Source: CAD feature listing. Evaluate the final solid. Frame: model axes, mm. A direction names the side the tool comes from. Round coordinates to 2 decimals unless told otherwise and drop trailing zeros. Order: outer loops, then holes, each group sorted by start corner. A loop starts at its lowest first (then second) coordinate and runs counter-clockwise, first axis right, second up. Notation, with made-up numbers: M 60.5,57 L 94.5,57 A14 ccw 94.5,79 Z; hole C -36,-16.75 d7. An arc over 180 degrees is marked long. Use CSV: the item, a comma, the result in double quotes. Start each with the question number.
```python
from build123d import *

# Parameters (mm, degrees)
SKETCH1_W           = 24
SKETCH1_H           = 90
BOSS_EXTRUDE1_DEPTH = 20
CUT_EXTRUDE1_DEPTH  = 16
CUT_EXTRUDE8_DEPTH  = 10
FILLET1_R           = 20
SKETCH12_R          = 2.5
CUT_EXTRUDE9_DEPTH  = 18.5
SKETCH13_R          = 4.5
CUT_EXTRUDE10_DEPTH = 16.5
FILLET2_R           = 3
CHAMFER1_SIZE       = 3


with BuildPart() as part:
    # Sketch1 → Boss-Extrude1 (new body)
    with BuildSketch(Plane.XY):
        with Locations((12, 45)):
            Rectangle(SKETCH1_W, SKETCH1_H)
    extrude(amount=-BOSS_EXTRUDE1_DEPTH)

    # Sketch4 → Cut-Extrude1 (cut)
    with BuildSketch(Plane.XY):
        Polygon((20.5, 83), (18.5, 83), (18.5, 61), (19.5, 61), (8, 15), (8, 0), (24, 0), (24, 90), (20.5, 90), align=None)
    extrude(amount=-CUT_EXTRUDE1_DEPTH, mode=Mode.SUBTRACT)

    # Sketch9 → Cut-Extrude8 (cut)
    with BuildSketch(Plane(origin=(0, 0, -20), x_dir=(-1, 0, 0), z_dir=(0, 0, -1))):
        Polygon((-24, 0), (-24, 45), (-8, 15), (-8, 0), align=None)
    extrude(amount=-CUT_EXTRUDE8_DEPTH, mode=Mode.SUBTRACT)

    # Fillet1
    fillet1_edges = [part.edges().sort_by_distance(p)[0] for p in [
        (24, 45, -18),
    ]]
    fillet(fillet1_edges, radius=FILLET1_R)

    # Sketch12 → Cut-Extrude9 (cut)
    with BuildSketch(Plane(origin=(18.5, 0, 0), x_dir=(0, 0, -1), z_dir=(1, 0, 0))):
        with Locations(Location((10, 72, 0), (0, 0, 90))):
            Circle(SKETCH12_R)
        with Locations(Location((10, 7.5, 0), (0, 0, 90))):
            Circle(SKETCH12_R)
    extrude(amount=-CUT_EXTRUDE9_DEPTH, mode=Mode.SUBTRACT)

    # Sketch13 → Cut-Extrude10 (cut)
    with BuildSketch(Plane(origin=(18.5, 0, 0), x_dir=(0, 0, -1), z_dir=(1, 0, 0))):
        with Locations(Location((10, 72, 0), (0, 0, 90))):
            Circle(SKETCH13_R)
        with Locations(Location((10, 7.5, 0), (0, 0, 90))):
            Circle(SKETCH13_R)
    extrude(amount=-CUT_EXTRUDE10_DEPTH, mode=Mode.SUBTRACT)

    # Fillet2
    # the kernel refuses this fillet: 3 mm, written as the material it takes off along each edge
    with BuildSketch(Plane(origin=(0, 90, 7.5), x_dir=(1, 0, 0), z_dir=(0, 0, -1)), Plane(origin=(8, 0, -27.5), x_dir=(0, 1, 0), z_dir=(0, 0, 1)), Plane(origin=(0, 0, 7.5), x_dir=(0, 1, 0), z_dir=(0, 0, -1))) as fillet2_piece_1:
        with BuildLine():
            CenterArc((FILLET2_R, FILLET2_R), FILLET2_R, 180, 90)
            Line((0, FILLET2_R), (-FILLET2_R * 0.02, FILLET2_R))
            Line((-FILLET2_R * 0.02, FILLET2_R), (-FILLET2_R * 0.02, -FILLET2_R * 0.02))
            Line((-FILLET2_R * 0.02, -FILLET2_R * 0.02), (FILLET2_R, -FILLET2_R * 0.02))
            Line((FILLET2_R, -FILLET2_R * 0.02), (FILLET2_R, 0))
        make_face()
    extrude(amount=35, mode=Mode.SUBTRACT)
    with BuildSketch(Plane(origin=(24, 90, -8.5), x_dir=(0, -1, 0), z_dir=(0, 0, -1))) as fillet2_piece_2:
        with BuildLine():
            CenterArc((FILLET2_R, FILLET2_R), FILLET2_R, 180, 90)
            Line((0, FILLET2_R), (-FILLET2_R * 0.02, FILLET2_R))
            Line((-FILLET2_R * 0.02, FILLET2_R), (-FILLET2_R * 0.02, -FILLET2_R * 0.02))
            Line((-FILLET2_R * 0.02, -FILLET2_R * 0.02), (FILLET2_R, -FILLET2_R * 0.02))
            Line((FILLET2_R, -FILLET2_R * 0.02), (FILLET2_R, 0))
        make_face()
    extrude(amount=19, mode=Mode.SUBTRACT)
    with BuildSketch(Plane(origin=(19.5, 61, 6.128837665), x_dir=(-0.24253562503633366, -0.9701425001453317, 0), z_dir=(0, 0, -1))) as fillet2_piece_3:
        with BuildLine():
            CenterArc((2.451535066, 3), FILLET2_R, 222.580014358, 47.419985642)
            Line((0.242535625, 0.9701425), (0.198355636, 0.92954535))
            ThreePointArc((0.198355636, 0.92954535), (0.063059263, 0.499623388), (-0.05820855, 0.014552138))
            Line((-0.05820855, 0.014552138), (0, -0.06))
            Line((0, -0.06), (2.451535066, -0.06))
            Line((2.451535066, -0.06), (2.451535066, 0))
        make_face()
    extrude(amount=22.128837665, mode=Mode.SUBTRACT)

    # Chamfer1
    # the kernel refuses this chamfer: 3 mm, written as the material it takes off along each edge
    with BuildSketch(Plane(origin=(21, 87, -16), x_dir=(1, 0, 0), z_dir=(0, -1, 0))) as chamfer1_piece_1:
        Polygon((3 - CHAMFER1_SIZE, 0), (3, -CHAMFER1_SIZE), (3, 0), align=None)
    revolve(axis=Axis((21, 87, -16), (0, 0, 1)), revolution_arc=90, mode=Mode.SUBTRACT)
    with BuildSketch(Plane(origin=(24, 50, -16), x_dir=(-1, 0, 0), z_dir=(0, 1, 0))) as chamfer1_piece_2:
        Polygon((CHAMFER1_SIZE, 0), (0, -CHAMFER1_SIZE), (0, 0), align=None)
    extrude(amount=37, mode=Mode.SUBTRACT)
    with BuildSketch(Plane(origin=(4.369388723, 8.192603855, -16), x_dir=(0, 0, -1), z_dir=(0.47058823529411764, 0.8823529411764706, 0))) as chamfer1_piece_3_section:
        Polygon((CHAMFER1_SIZE, 0), (0, CHAMFER1_SIZE), (0, 0), align=None)
    chamfer1_piece_3 = extrude(amount=36.715048964, mode=Mode.PRIVATE)
    chamfer1_piece_3 = split(chamfer1_piece_3, bisect_by=Plane(origin=(8, 8.192603855, -16), z_dir=(1, 0, 0)), keep=Keep.TOP, mode=Mode.PRIVATE)
    chamfer1_piece_3 = split(chamfer1_piece_3, bisect_by=Plane(origin=(6.184694361, 7.738777446, -16), z_dir=(0.9701425001453319, -0.24253562503633322, 0)), keep=Keep.TOP, mode=Mode.PRIVATE)
    add(chamfer1_piece_3, mode=Mode.SUBTRACT)
    with BuildSketch(Plane(origin=(4, 50, -16), x_dir=(0.8823529411764705, -0.47058823529411764, 0), z_dir=(-0.47058823529411764, -0.8823529411764705, 0))) as chamfer1_piece_4:
        Polygon((20, -CHAMFER1_SIZE), (20 - CHAMFER1_SIZE, 0), (20, 0), align=None)
    revolve(axis=Axis((4, 50, -16), (0, 0, 1)), revolution_arc=28.072486936, mode=Mode.SUBTRACT)
    with BuildSketch(Plane(origin=(21, 90, -16), x_dir=(0, -1, 0), z_dir=(-1, 0, 0))) as chamfer1_piece_5:
        Polygon((CHAMFER1_SIZE, 0), (0, -CHAMFER1_SIZE), (0, 0), align=None)
    extrude(amount=0.5, mode=Mode.SUBTRACT)


solid = part.part
```
(1) Section B-B on z = -2. Return loops of the section in (x, y).
(2) Draft query along Y for faces 1 (the face through (23.386, 45.083, -19.493)), 2 (the face through (20.8, 88.5, -17.5)), 3 (the face through (5.042, 11.792, -8.648)). Return one class per face: pulls with the +Y half, pulls with the -Y half, needs draft (parallel to the pull), parting line crosses it, or undercut.
(3) Reachability of faces 4 (the face through (18.5, 75, -6)), 5 (the face through (13.376, 36.505, -9.367)), 6 (the face through (2, 9.4, -11.9)) from +Z, -Z, +X, -X, +Y, -Y: full face, straight path, thin tool, end or side. Return the list, or none.
(4) Section D-D on x = 9.25. Return loops of the section in (y, z), plus the area to 3 significant figures.
(5) Contact query for flat-ended pins moving along their axis: P1, Ø1, axis at y = 43, z = -4.5, coming from the +X side (3 decimals); P2, Ø5.5, axis at y = 72, z = -10, coming from the +X side; P3, Ø7.5, axis at y = 86.5, z = -10.5, coming from the +X side. Output: stop coordinate, or through.
(6) Section C-C on y = 7.5. Return loops of the section in (x, z), plus the area to 3 significant figures.
(7) Section A-A on y = 72. Return loops of the section in (x, z), plus the area to 3 significant figures.
(8) Line query: line 1 along Z through (x, y) = (1.5, 72); line 2 along Z through (x, y) = (6.8, 7.5); line 3 along Z through (x, y) = (19, 60). Output: solid intervals per line, ascending.
Results below:
1,outline,"M 0,3 A3 ccw 3,0 L 5,0 A3 ccw 8,3 L 8,15 L 18.91,58.62 A3 ccw 18.5,61 L 18.5,83 L 20.5,83 L 20.5,90 L 3,90 A3 ccw 0,87 Z"
2,face 1,"pulls with the -Y half"
2,face 2,"pulls with the +Y half"
2,face 3,"undercut"
3,face 4,"+Z, +X"
3,face 5,"+Z, +X, -Y"
3,face 6,"+X"
4,outline,"M 17.34,-20 L 90,-20 L 90,0 L 20,0 L 20,-17.75 L 17.34,-19 Z; hole C 72,-10 d9"
4,area,"1,340 mm2"
5,P1,"stops at x = 15.125"
5,P2,"stops at x = 2"
5,P3,"stops at x = 20.5"
6,outline,"M 0,-20 L 8,-20 L 8,-14.5 L 2,-14.5 L 2,-12.5 L 0,-12.5 Z; M 0,-7.5 L 2,-7.5 L 2,-5.5 L 8,-5.5 L 8,0 L 0,0 Z"
6,area,"96.0 mm2"
7,outline,"M 0,-20 L 24,-20 L 24,-19 L 21,-16 L 18.5,-16 L 18.5,-14.5 L 2,-14.5 L 2,-12.5 L 0,-12.5 Z; M 0,-7.5 L 2,-7.5 L 2,-5.5 L 18.5,-5.5 L 18.5,0 L 0,0 Z"
7,area,"229 mm2"
8,line 1,"z = -20 to -12.5, -7.5 to 0"
8,line 2,"z = -20 to -14.5, -5.5 to 0"
8,line 3,"z = -20 to -16"
